Check sheet for the modelled part. Datum: model origin and axes. Units: mm. Give positions to 0.01 mm unless a question says otherwise; leave off trailing zeros. Loops run counter-clockwise (first coordinate to the right, second up) from the corner with the lowest first, then second, coordinate; pieces in that order, holes last. Notation, with made-up numbers: (65.5, -25) -> (83.5, -25) arc R33 ccw to (83.5, 14) -> close; hole circle Ø4 at (20, -38.5). An arc over 180 degrees is marked (long way). Answer as CSV lines item,"result". Start each with the question number.
(1) Release check for a two-part mould opening along Y. For faces 1 (the face through (2.03, -24.3, -56.93)), 2 (the face through (2, 82, -15.625)) record: pulls with the +Y half, pulls with the -Y half, needs draft (parallel to the pull), parting line crosses it, or undercut.
(2) Section check C-C on x = 3.4. State how many separate pieces and enclosed holes the cut face has, plus the area to 3 significant figures.
(3) Section check D-D on z = 37.5. Enter the section's corners in (x, y).
(4) Material ranges on line 1 (Y direction, x = 0.6, z = -12); line 2 (Y direction, x = 2, z = -1.5); line 3 (Z direction, x = 2.3, y = -2.5) (3 decimals), recorded low to high. Write a range as from..to.
(5) Section check B-B on z = -13.5. Enter the section's corners in (x, y).
(6) Section check A-A on y = 6. Enter the section's corners in (x, z).
(7) Gauge pin test, flat ends, axial feed: pin 1 Ø1.2 at (x, y) = (1.5, 82) entering from +Z; pin 2 Ø8 at (y, z) = (-21, 11.5) entering from -X; pin 3 Ø2 at (x, z) = (2, -54.5) entering from -Y. Record the tip position at first contact, or that the pin passes through.
from build123d import *

# Parameters (mm, degrees)
SCHIZZO1_W                   = 50
SCHIZZO1_H                   = 80
ESTRUSIONE_ESTRUSIONE1_DEPTH = 4
SCHIZZO2_W                   = 4
SCHIZZO2_H                   = 2.857142857
SCHIZZO2_W_2                 = 7
ESTRUSIONE_ESTRUSIONE2_DEPTH = 4
SCHIZZO3_W                   = 4
SCHIZZO3_H                   = 5.714285715
SCHIZZO3_W_2                 = 7
ESTRUSIONE_ESTRUSIONE3_DEPTH = 4
RIPETIZIONE_A_L1_COUNT       = 6
RIPETIZIONE_A_L1_PITCH       = 11.428571
SCHIZZO4_W                   = 6.25
SCHIZZO4_H                   = 4
ESTRUSIONE_ESTRUSIONE4_DEPTH = 4
RIPETIZIONE_A_L2_COUNT       = 4
RIPETIZIONE_A_L2_PITCH       = 12.5
SCHIZZO5_W                   = 61
SCHIZZO5_H                   = 88
ESTRUSIONE_ESTRUSIONE5_DEPTH = 4
RACCORDO1_R                  = 10
RACCORDO2_R                  = 10


with BuildPart() as part:
    # Schizzo1 → Estrusione-Estrusione1 (new body)
    with BuildSketch(Plane(origin=(0, 0, 0), x_dir=(0, 0, -1), z_dir=(1, 0, 0))):
        with Locations((25, 40)):
            Rectangle(SCHIZZO1_W, SCHIZZO1_H)
    extrude(amount=ESTRUSIONE_ESTRUSIONE1_DEPTH)

    # Schizzo2 → Estrusione-Estrusione2 (add)
    with BuildSketch(Plane(origin=(4, 0, 0), x_dir=(0, 0, -1), z_dir=(1, 0, 0))):
        with Locations((-2, 78.571428572)):
            Rectangle(SCHIZZO2_W, SCHIZZO2_H)
        with Locations((53.5, 78.571428572)):
            Rectangle(SCHIZZO2_W_2, SCHIZZO2_H)
        with Locations((53.5, 1.428571429)):
            Rectangle(SCHIZZO2_W_2, SCHIZZO2_H)
        with Locations((-2, 1.428571429)):
            Rectangle(SCHIZZO2_W, SCHIZZO2_H)
    extrude(amount=-ESTRUSIONE_ESTRUSIONE2_DEPTH)

    # Schizzo3 → Estrusione-Estrusione3 (add)
    with BuildSketch(Plane(origin=(4, 0, 0), x_dir=(0, 0, -1), z_dir=(1, 0, 0))):
        with Locations((-2, 68.571428572)):
            Rectangle(SCHIZZO3_W, SCHIZZO3_H)
        with Locations((53.5, 68.571428572)):
            Rectangle(SCHIZZO3_W_2, SCHIZZO3_H)
    estrusione_estrusione3 = extrude(amount=-ESTRUSIONE_ESTRUSIONE3_DEPTH)

    # Ripetizione a L1: Estrusione-Estrusione3 ×6
    with Locations(*[(0, -i * RIPETIZIONE_A_L1_PITCH, 0) for i in range(1, RIPETIZIONE_A_L1_COUNT)]):
        add(estrusione_estrusione3)

    # Schizzo4 → Estrusione-Estrusione4 (add)
    with BuildSketch(Plane(origin=(4, 0, 0), x_dir=(0, 0, -1), z_dir=(1, 0, 0))):
        with Locations((6.25, 82)):
            Rectangle(SCHIZZO4_W, SCHIZZO4_H)
        with Locations((6.25, -2)):
            Rectangle(SCHIZZO4_W, SCHIZZO4_H)
    estrusione_estrusione4 = extrude(amount=-ESTRUSIONE_ESTRUSIONE4_DEPTH)

    # Ripetizione a L2: Estrusione-Estrusione4 ×4
    with Locations(*[(0, 0, -i * RIPETIZIONE_A_L2_PITCH) for i in range(1, RIPETIZIONE_A_L2_COUNT)]):
        add(estrusione_estrusione4)

    # Schizzo5 → Estrusione-Estrusione5 (add)
    with BuildSketch(Plane(origin=(4, 0, 0), x_dir=(0, 0, -1), z_dir=(1, 0, 0))):
        Polygon((64, -11), (46.160080614, -44.552008529), (-54.590569466, 9.018062365), (-11, 91), (64, 91), align=None)
        with Locations((26.5, 40)):
            Rectangle(SCHIZZO5_W, SCHIZZO5_H, mode=Mode.SUBTRACT)
    extrude(amount=-ESTRUSIONE_ESTRUSIONE5_DEPTH)

    # Raccordo1
    raccordo1_edges = [part.edges().sort_by_distance(p)[0] for p in [
        (2, -44.552008529, -46.160080614),
        (2, 9.018062365, 54.590569466),
    ]]
    fillet(raccordo1_edges, radius=RACCORDO1_R)

    # Raccordo2
    raccordo2_edges = [part.edges().sort_by_distance(p)[0] for p in [
        (2, 91, -64),
        (2, -11, -64),
        (2, 91, 11),
    ]]
    fillet(raccordo2_edges, radius=RACCORDO2_R)


solid = part.part
Working result:
1,face 1,"pulls with the -Y half"
1,face 2,"undercut"
2,separate pieces,"1"
2,enclosed holes,"24"
2,area,"10,500 mm^2"
3,outline,"(0, -0.07) -> (4, -0.07) -> (4, 41.16) -> (0, 41.16) -> close"
4,line 1,"y = -26.39..-4, 0..80, 84..91"
4,line 2,"y = -20.81..-4, 0..80, 84..91"
4,line 3,"z = -64..-57, -46.875..-40.625, -34.375..-28.125, -21.875..-15.625, -9.375..-3.125, 4..32.928"
5,outline,"(0, -27.19) -> (4, -27.19) -> (4, -4) -> (0, -4) -> close; (0, 0) -> (4, 0) -> (4, 80) -> (0, 80) -> close; (0, 84) -> (4, 84) -> (4, 91) -> (0, 91) -> close"
6,outline,"(0, -64) -> (4, -64) -> (4, -57) -> (0, -57) -> close; (0, -50) -> (4, -50) -> (4, 0) -> (0, 0) -> close; (0, 4) -> (4, 4) -> (4, 48.05) -> (0, 48.05) -> close"
7,pin 1,"stops at z = 16.1"
7,pin 2,"passes through"
7,pin 3,"stops at y = -30.75"
